Can you work these out from the model? Positions are in its coordinate system, mm. Face numbers are marked on the shaded views. A direction names the side the tool comes from. Round coordinates to 2 decimals unless told otherwise and drop trailing zeros. Write each loop counter-clockwise with the first axis right and the second up, starting at its lowest first coordinate (ties: lowest second). Pieces come first, ordered by that corner, then holes. Notation, with made-up numbers: M 67,2 L 103,2 A11 cw 103,20 Z; hole C 61,87 d2. An arc over 180 degrees is marked long. Answer as a JSON object with one key per item and string values. Group by question number.
1) Please list where these lines run through material, in increasing order: L1, parallel to X at y = -1.5, z = 22; L2, parallel to Z at x = 34.5, y = -12.5; L3, parallel to Z at x = 5.5, y = -13. Write a range as [from, to].
2) I'm going to push flat-ended pins straight in: pin 1 Ø12 at (x, z) = (37, 26.5) entering from -Y; pin 2 Ø16.5 at (x, y) = (27, -9) entering from +Z. Where does each tip first touch, or does it pass through?
3) Suppose I cut it at D-D, the plane z = 33.5. Write out the boundary of the cut face in (x, y).
4) On a 3-axis mill with a long thin cutter (end or side, diameter ignored), from which of +Z, -Z, +X, -X, +Y, -Y can I reach the whole of each face in a straight line? I mean the marked faces 4 and 5. Say none if no direction works.
5) If we mould it in two halves opening along X, with no side actions, what happens to the marked faces 1, 2 and 3? For each: +X half, -X half, draft (parallel to the pull), parting line (faces both ways), or undercut.
6) Suppose I cut it at A-A, the plane z = 24. Write out the boundary of the cut face in (x, y).
7) Suppose I cut it at C-C, the plane y = -8. Write out the boundary of the cut face in (x, z).
8) Suppose I cut it at B-B, the plane x = 27. Write out the boundary of the cut face in (y, z).
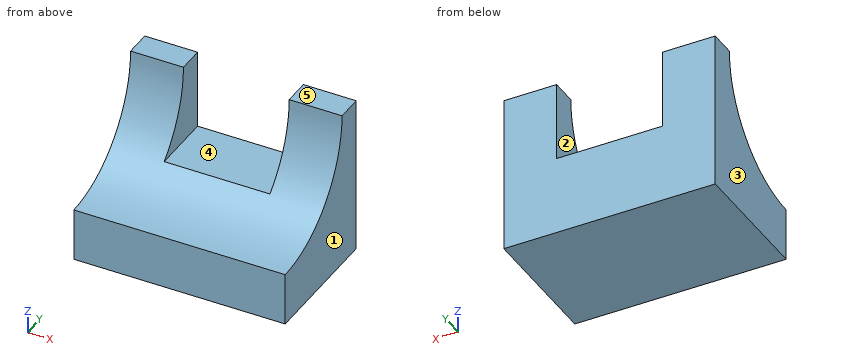
from build123d import *

# Parameters (mm, degrees)
F0_W     = 50.8
F0_H     = 38.1
F1_DEPTH = 31.75
F2_W     = 25.4
F2_H     = 19.05
F3_DEPTH = 31.751
F5_DEPTH = 50.8


with BuildPart() as f1:
    # F0 (on Front) → F1 (new body)
    with BuildSketch(Plane.XZ):
        with Locations((25.4, 19.05)):
            Rectangle(F0_W, F0_H)
    extrude(amount=F1_DEPTH)

    # F2 (on face) → F3 (cut, through all)
    with BuildSketch(Plane.XZ.offset(31.75)):
        with Locations((25.4, 28.575)):
            Rectangle(F2_W, F2_H)
    extrude(amount=-F3_DEPTH, mode=Mode.SUBTRACT)

    # F4 (on face) → F5 (cut)
    with BuildSketch(Plane.YZ.offset(50.8)):
        with BuildLine():
            ThreePointArc((-31.75, 12.7), (-13.789488, 20.139488), (-6.35, 38.1))
            Line((-6.35, 38.1), (-31.75, 38.1))
            Line((-31.75, 38.1), (-31.75, 12.7))
        make_face()
        with BuildLine():
            Line((-31.75, 38.1), (-6.35, 38.1))
            ThreePointArc((-6.35, 38.1), (-49.710512, 56.060512), (-31.75, 12.7))
            Line((-31.75, 12.7), (-31.75, 38.1))
        make_face()
    extrude(amount=-F5_DEPTH, mode=Mode.SUBTRACT)


solid = f1.part
Results:
{
 "1": {"L1": "[0, 12.7], [38.1, 50.8]", "L2": "[0, 19.05]", "L3": "[0, 20.97]"},
 "2": {"pin 1": "y = -13.34", "pin 2": "z = 19.05"},
 "3": {"outline": "M 0,-6.77 L 12.7,-6.77 L 12.7,0 L 0,0 Z; M 38.1,-6.77 L 50.8,-6.77 L 50.8,0 L 38.1,0 Z"},
 "4": {"face 4": "+Z, +Y, -Y", "face 5": "+Z, +X, -X, +Y, -Y"},
 "5": {"face 1": "+X half", "face 2": "undercut", "face 3": "-X half"},
 "6": {"outline": "M 0,-10.62 L 12.7,-10.62 L 12.7,0 L 0,0 Z; M 38.1,-10.62 L 50.8,-10.62 L 50.8,0 L 38.1,0 Z"},
 "7": {"outline": "M 0,0 L 50.8,0 L 50.8,29.09 L 38.1,29.09 L 38.1,19.05 L 12.7,19.05 L 12.7,29.09 L 0,29.09 Z"},
 "8": {"outline": "M -31.75,0 L 0,0 L 0,19.05 L -14.95,19.05 A25.4 cw -31.75,12.7 Z"}
}
